from build123d import *

# Parameters (mm, degrees)
SKETCH102_W      = 5
SKETCH102_H      = 4
EXTRUDE093_DEPTH = 5
EXTRUDE064_DEPTH = 25


with BuildPart() as extrude093:
    # Sketch102 → Extrude093 (new body)
    with BuildSketch(Plane(origin=(-6, 0, 0), x_dir=(0, -1, 0), z_dir=(-1, 0, 0))):
        with Locations((-89, 2)):
            Rectangle(SKETCH102_W, SKETCH102_H)
    extrude(amount=-EXTRUDE093_DEPTH)


with BuildPart() as cut015:
    # Sketch074 → Extrude064 (new body)
    with BuildSketch(Plane.XY.offset(3)):
        Polygon((-4, 93.5), (0, 93.5), (0, 92), (-2.5, 92), (-2.5, 10.5), (0, 10.5), (0, 9), (-4, 9), align=None)
    extrude(amount=-EXTRUDE064_DEPTH)

    # Cut015: cut Extrude093
    add(extrude093.part, mode=Mode.SUBTRACT)


solid = cut015.part
Could you check a few things on this model? Use its own coordinates, in mm. A direction names the side the tool comes from. Coordinates: 2 decimals unless noted, no trailing zeros. Write each loop counter-clockwise with the first axis right and the second up, starting at its lowest first coordinate (ties: lowest second). Pieces come first, ordered by that corner, then holes. Notation, with made-up numbers: (67.25, 25) - (91.25, 25) arc R12 cw to (91.25, 43) - close; hole circle Ø10 at (-13.75, 36). An arc over 180 degrees is marked (long way). Write item = value, one per line.
1) Suppose I cut it at A-A on x = -1.1. Please give me the cut outline in (y, z).
Result set:
outline = (9, -22) - (10.5, -22) - (10.5, 3) - (9, 3) - close; (92, -22) - (93.5, -22) - (93.5, 3) - (92, 3) - close
2) Please list where these lines run through material, in increasing order: line 1 (Y direction, x = -3.2, z = 1.25); line 2 (Y direction, x = -0.75, z = 1); line 3 (X direction, y = 13, z = -11). Write a range as [from, to].
Result set:
line_1 = [9, 86.5], [91.5, 93.5]
line_2 = [9, 10.5], [92, 93.5]
line_3 = [-4, -2.5]
3) Suppose I cut it at C-C on y = 70. Please give me the cut outline in (x, z), plus the area to 3 significant figures.
Result set:
outline = (-4, -22) - (-2.5, -22) - (-2.5, 3) - (-4, 3) - close
area = 37.5 mm2
4) For faces 5 (the flat face through (0, 93, -9)), 6 (the flat face through (-1, 92, -9)), 7 (the flat face through (-3, 86.5, 1)), which set-ups out of +Z, -Z, +X, -X, +Y, -Y let a thin tool reach every point of the face, with its end or its side?
Result set:
face_5 = +Z, -Z, +X, +Y, -Y
face_6 = +Z, -Z, +X
face_7 = +Z, +X, -X
5) We'd pull the mould along Y, two halves only. Please class faces 1 (the flat face through (-4, 51, -9)), 2 (the flat face through (-2, 9, -9)), 3 (the flat face through (-3, 91.5, 1)), 4 (the flat face through (-2, 93.5, -9)): +Y half, -Y half, draft (parallel to the pull), parting line (faces both ways), or undercut.
Result set:
face_1 = draft
face_2 = -Y half
face_3 = undercut
face_4 = +Y half
6) Suppose I cut it at B-B on z = -7.75. Please give me the cut outline in (x, y), plus the area to 3 significant figures.
Result set:
outline = (-4, 9) - (0, 9) - (0, 10.5) - (-2.5, 10.5) - (-2.5, 92) - (0, 92) - (0, 93.5) - (-4, 93.5) - close
area = 134 mm2
7) Will these pins go through, and if not, where does the flat tip stop? pin 1 Ø2 at (y, z) = (44.5, -17.5) entering from +X; pin 2 Ø1.2 at (x, y) = (-3.5, 88.5) entering from +Z.
Result set:
pin_1 = -2.5
pin_2 = 0
